Verification items for the finished model (mm, model axes). A direction names the side the tool comes from. Give positions to 0.01 mm unless a question says otherwise; leave off trailing zeros. Write each loop counter-clockwise with the first axis right and the second up, starting at its lowest first coordinate (ties: lowest second). Pieces come first, ordered by that corner, then holes.
from build123d import *

# Parameters (mm, degrees)
F1_DEPTH = 12.7
F2_DEPTH = 76.2
F3_R     = 12.7
F3_R_2   = 7.112
F4_DEPTH = 9.2456
F5_DEPTH = 38.101
F3_W     = 31.75
F3_H     = 7.874
F6_DEPTH = 38.101
F7_W     = 63.5
F7_H     = 25.4
F8_DEPTH = 63.501


with BuildPart() as f1:
    # F0 (on Right) → F1 (new body)
    with BuildSketch(Plane.YZ):
        with BuildLine():
            Line((0, 60.452), (0, 38.1))
            Line((0, 38.1), (63.5, 38.1))
            Line((63.5, 38.1), (63.5, 60.452))
            ThreePointArc((63.5, 60.452), (59.780256, 69.432256), (50.8, 73.152))
            Line((50.8, 73.152), (12.7, 73.152))
            ThreePointArc((12.7, 73.152), (3.719744, 69.432256), (0, 60.452))
        make_face()
        with BuildLine():
            ThreePointArc((12.7, 52.578), (4.826, 60.452), (12.7, 68.326))
            Line((12.7, 68.326), (50.8, 68.326))
            ThreePointArc((50.8, 68.326), (58.674, 60.452), (50.8, 52.578))
            Line((50.8, 52.578), (12.7, 52.578))
        make_face(mode=Mode.SUBTRACT)
    extrude(amount=F1_DEPTH)

    # F0 (on Right) → F2 (join)
    with BuildSketch(Plane.YZ):
        Polygon((0, 38.1), (0, 0), (8.423471, 0), (8.423471, 6.35), (55.076529, 6.35), (55.076529, 0), (63.5, 0), (63.5, 38.1), align=None)
    extrude(amount=F2_DEPTH)

    # F3 (on face) → F4 (cut)
    with BuildSketch(Plane.XY.offset(38.1)):
        with Locations((44.45, 31.75)):
            Circle(F3_R)
        with Locations((44.45, 31.75)):
            Circle(F3_R_2, mode=Mode.SUBTRACT)
    extrude(amount=-F4_DEPTH, mode=Mode.SUBTRACT)

    # F3 (on face) → F5 (cut, through all)
    with BuildSketch(Plane.XY.offset(38.1)):
        with Locations((44.45, 31.75)):
            Circle(F3_R_2)
    extrude(amount=-F5_DEPTH, mode=Mode.SUBTRACT)

    # F3 (on face) → F6 (cut, through all)
    with BuildSketch(Plane.XY.offset(38.1)):
        with Locations((44.45, 59.563)):
            Rectangle(F3_W, F3_H)
        with Locations((44.45, 3.937)):
            Rectangle(F3_W, F3_H)
    extrude(amount=-F6_DEPTH, mode=Mode.SUBTRACT)

    # F7 (on face) → F8 (cut, through all)
    with BuildSketch(Plane.XZ):
        with Locations((31.75, 12.7)):
            Rectangle(F7_W, F7_H)
    extrude(amount=-F8_DEPTH, mode=Mode.SUBTRACT)


solid = f1.part
Item 1: Depth check by flat-ended pin: pin 1 (6.5 mm diameter, centred on y = 5.5, z = 31.5, fed in from -X); pin 2 (2 mm diameter, centred on x = 37, y = 25, fed in from +Z); pin 3 (4 mm diameter, centred on x = 47, z = 31, fed in from +Y); pin 4 (6 mm diameter, centred on x = 50, y = 11.5, fed in from +Z). Enter the tip coordinate at first touch or a pass-through.
Answer key:
pin 1: stops at x = 0
pin 2: stops at z = 28.85
pin 3: stops at y = 55.63
pin 4: stops at z = 38.1
Item 2: Sectioned sample at A-A on x = 44.45. Record the cut outline in (y, z).
Answer key:
outline: (7.87, 25.4) - (24.64, 25.4) - (24.64, 28.85) - (19.05, 28.85) - (19.05, 38.1) - (7.87, 38.1) - close; (38.86, 25.4) - (55.63, 25.4) - (55.63, 38.1) - (44.45, 38.1) - (44.45, 28.85) - (38.86, 28.85) - close
Item 3: Sectioned sample at D-D on z = 57. Record the cut outline in (x, y), then the cut area to 3 significant figures.
Answer key:
outline: (0, 0) - (12.7, 0) - (12.7, 5.62) - (0, 5.62) - close; (0, 57.88) - (12.7, 57.88) - (12.7, 63.5) - (0, 63.5) - close
area: 143 mm2
Item 4: Set-up check for faces 1 (the face through (70, 55.077, 3)), 2 (the face through (28.575, 4, 32)), 3 (the face through (50, 26, 28.854)), 4 (the face through (6, 31, 68.326)): record each of +Z, -Z, +X, -X, +Y, -Y from which the full face is reachable in a straight line by a thin tool's end or side.
Answer key:
face 1: -Z, +X, -X
face 2: +Z, -Z, -Y
face 3: +Z
face 4: +X, -X
Item 5: Scan lines: line 1 along X through (y, z) = (31, 32); line 2 along Z through (x, y) = (8, 29.5); line 3 along X through (y, z) = (41.5, 19). Record each from-to range of solid material in increasing order.
Answer key:
line 1: x = 0 to 31.77, 57.13 to 76.2
line 2: z = 25.4 to 52.58, 68.33 to 73.15
line 3: x = 63.5 to 76.2
Item 6: Release check for a two-part mould opening along Z. For faces 5 (the face through (31, 31, 25.4)), 6 (the face through (6.26, 58.67, 60.63)), 7 (the face through (63.5, 31, 15)) record: released by +Z, released by -Z, zero draft, split by the parting line, or undercut.
Answer key:
face 5: released by -Z
face 6: undercut
face 7: zero draft
Item 7: Sectioned sample at C-C on x = 7.5. Record the cut outline in (y, z).
Answer key:
outline: (0, 25.4) - (63.5, 25.4) - (63.5, 60.45) arc R12.7 ccw to (50.8, 73.15) - (12.7, 73.15) arc R12.7 ccw to (0, 60.45) - close; hole (12.7, 52.58) - (50.8, 52.58) arc R7.87 ccw to (50.8, 68.33) - (12.7, 68.33) arc R7.87 ccw to start
Item 8: Sectioned sample at B-B on y = 31.75. Record the cut outline in (x, z).
Answer key:
outline: (0, 25.4) - (37.34, 25.4) - (37.34, 28.85) - (31.75, 28.85) - (31.75, 38.1) - (12.7, 38.1) - (12.7, 52.58) - (0, 52.58) - close; (0, 68.33) - (12.7, 68.33) - (12.7, 73.15) - (0, 73.15) - close; (51.56, 25.4) - (63.5, 25.4) - (63.5, 6.35) - (76.2, 6.35) - (76.2, 38.1) - (57.15, 38.1) - (57.15, 28.85) - (51.56, 28.85) - close
